from build123d import *

# Parameters (mm, degrees)
SKETCH1_W                                = 152.4
SKETCH1_H                                = 101.6
BOSS_EXTRUDE1_DEPTH                      = 12.7
CBORE_FOR_3_8_HEX_HEAD_BOLT1_D           = 10.0838
CBORE_FOR_3_8_HEX_HEAD_BOLT1_CBORE_D     = 22.225
CBORE_FOR_3_8_HEX_HEAD_BOLT1_CBORE_DEPTH = 6.35
F_1_4_0_25_DIAMETER_HOLE2_D              = 6.858
CUT_EXTRUDE1_DEPTH                       = 6.35


with BuildPart() as part:
    # Sketch1 → Boss-Extrude1 (new body)
    with BuildSketch(Plane(origin=(0, 0, 0), x_dir=(1, 0, 0), z_dir=(0, 1, 0))):
        Rectangle(SKETCH1_W, SKETCH1_H)
    extrude(amount=BOSS_EXTRUDE1_DEPTH)

    # CBORE for 3/8 Hex Head Bolt1 (through all)
    with Locations(Plane(origin=(0, 12.7, 0), x_dir=(1, 0, 0), z_dir=(0, 1, 0))):
        with Locations((-50.000000076, 0), (50.000000076, 0), (0, 0)):
            CounterBoreHole(CBORE_FOR_3_8_HEX_HEAD_BOLT1_D / 2, CBORE_FOR_3_8_HEX_HEAD_BOLT1_CBORE_D / 2, CBORE_FOR_3_8_HEX_HEAD_BOLT1_CBORE_DEPTH)

    # 1/4 (0.25) Diameter Hole2 (through all)
    with Locations(Plane.XZ):
        with Locations((-38.1, -38.1), (38.1, -38.1), (38.1, 38.1), (-38.1, 38.1)):
            Hole(F_1_4_0_25_DIAMETER_HOLE2_D / 2)

    # Sketch6 → Cut-Extrude1 (cut)
    with BuildSketch(Plane.XZ):
        Polygon((38.170015284, -31.757905082), (32.64259233, -34.868317526), (32.572577046, -41.210412444), (38.029984716, -44.442094918), (43.55740767, -41.331682474), (43.627422954, -34.989587556), align=None)
        Polygon((-38.203510193, -31.758363325), (-43.643773559, -35.018824119), (-43.540263366, -41.360460794), (-37.996489807, -44.441636675), (-32.556226441, -41.181175881), (-32.659736634, -34.839539206), align=None)
        Polygon((-38.214534968, 44.44144714), (-43.649121804, 41.171533378), (-43.534586835, 34.830086238), (-37.985465032, 31.75855286), (-32.550878196, 35.028466622), (-32.665413165, 41.369913762), align=None)
        Polygon((38.053503852, 44.44231095), (32.584149524, 41.23088863), (32.630645672, 34.88857768), (38.146496148, 31.75768905), (43.615850476, 34.96911137), (43.569354328, 41.31142232), align=None)
    extrude(amount=-CUT_EXTRUDE1_DEPTH, mode=Mode.SUBTRACT)


solid = part.part
Could you check a few things on this model? Use its own coordinates, in mm. A direction names the side the tool comes from. Coordinates: 2 decimals unless noted, no trailing zeros. Loops run counter-clockwise (first coordinate to the right, second up) from the corner with the lowest first, then second, coordinate; pieces in that order, holes last. Notation, with made-up numbers: (44, 50.25) -> (50, 50.25) arc R14 cw to (50, 68.25) -> close; hole circle Ø5 at (-2, 71.25). An arc over 180 degrees is marked (long way). Answer in a Markdown table with one row per item.
(1) If I drill on probe 1 along Z at (x, y) = (38.1, 9.75); probe 2 along Z at (x, y) = (-50, 9.5); probe 3 along Z at (x, y) = (-50, 3.5), over which ranges is the centre line in solid material (lowest first)?
Results found:
| item | result |
|---|---|
| probe 1 | z = -50.8 to -41.53, -34.67 to 34.67, 41.53 to 50.8 |
| probe 2 | z = -50.8 to -11.11, 11.11 to 50.8 |
| probe 3 | z = -50.8 to -5.04, 5.04 to 50.8 |
(2) Imagine slicing it at B-B (y = 9.75). List the corners of the cut face in (x, z) for me (1 decimal), plus the area to 3 significant figures.
Results found:
| item | result |
|---|---|
| outline | (-76.2, -50.8) -> (76.2, -50.8) -> (76.2, 50.8) -> (-76.2, 50.8) -> close; hole circle Ø22.2 at (-50, 0); hole circle Ø6.9 at (-38.1, -38.1); hole circle Ø6.9 at (-38.1, 38.1); hole circle Ø22.2 at (0, 0); hole circle Ø6.9 at (38.1, -38.1); hole circle Ø6.9 at (38.1, 38.1); hole circle Ø22.2 at (50, 0) |
| area | 14,200 mm^2 |
(3) Imagine slicing it at D-D (z = 38.1). List the corners of the cut face in (x, y) for me.
Results found:
| item | result |
|---|---|
| outline | (-76.2, 0) -> (-43.59, 0) -> (-43.59, 6.35) -> (-41.53, 6.35) -> (-41.53, 12.7) -> (-76.2, 12.7) -> close; (-34.67, 6.35) -> (-32.61, 6.35) -> (-32.61, 0) -> (32.61, 0) -> (32.61, 6.35) -> (34.67, 6.35) -> (34.67, 12.7) -> (-34.67, 12.7) -> close; (41.53, 6.35) -> (43.59, 6.35) -> (43.59, 0) -> (76.2, 0) -> (76.2, 12.7) -> (41.53, 12.7) -> close |
(4) For faces 1 (the face through (-35.573, 9.569, -35.783)), 2 (the face through (5, 6.35, 2)), 3 (the face through (-40.89, 3.13, 42.83)), which set-ups out of +Z, -Z, +X, -X, +Y, -Y let a thin tool reach every point of the face, with its end or its side?
Results found:
| item | result |
|---|---|
| face 1 | +Y, -Y |
| face 2 | +Y |
| face 3 | -Y |
(5) Imagine slicing it at A-A (x = 50). List the corners of the cut face in (y, z) for me, plus the area to 3 significant figures.
Results found:
| item | result |
|---|---|
| outline | (0, -50.8) -> (12.7, -50.8) -> (12.7, -11.11) -> (6.35, -11.11) -> (6.35, -5.04) -> (0, -5.04) -> close; (0, 5.04) -> (6.35, 5.04) -> (6.35, 11.11) -> (12.7, 11.11) -> (12.7, 50.8) -> (0, 50.8) -> close |
| area | 1,090 mm^2 |
(6) Imagine slicing it at C-C (z = 0). List the corners of the cut face in (x, y) for me.
Results found:
| item | result |
|---|---|
| outline | (-76.2, 0) -> (-55.04, 0) -> (-55.04, 6.35) -> (-61.11, 6.35) -> (-61.11, 12.7) -> (-76.2, 12.7) -> close; (-44.96, 0) -> (-5.04, 0) -> (-5.04, 6.35) -> (-11.11, 6.35) -> (-11.11, 12.7) -> (-38.89, 12.7) -> (-38.89, 6.35) -> (-44.96, 6.35) -> close; (5.04, 0) -> (44.96, 0) -> (44.96, 6.35) -> (38.89, 6.35) -> (38.89, 12.7) -> (11.11, 12.7) -> (11.11, 6.35) -> (5.04, 6.35) -> close; (55.04, 0) -> (76.2, 0) -> (76.2, 12.7) -> (61.11, 12.7) -> (61.11, 6.35) -> (55.04, 6.35) -> close |
(7) Thinking about a two-plate mould opening in Z: for faces 4 (the face through (-1, 12.7, -12)), 5 (the face through (-40.81, 3.13, -42.88)), which applies, released by +Z, released by -Z, zero draft, split by the parting line, or undercut?
Results found:
| item | result |
|---|---|
| face 4 | zero draft |
| face 5 | undercut |
(8) Will these pins go through, and if not, where does the flat tip stop? pin 1 Ø11 at (x, z) = (-47, -5) entering from +Y; pin 2 Ø11.5 at (x, z) = (-50, 0) entering from +Y; pin 3 Ø8 at (x, z) = (38.1, -38.1) entering from -Y.
Results found:
| item | result |
|---|---|
| pin 1 | stops at y = 12.7 |
| pin 2 | stops at y = 6.35 |
| pin 3 | stops at y = 6.35 |
